Can you work these out from the model? Positions are in its coordinate system, mm. A direction names the side the tool comes from. Give positions to 0.01 mm unless a question says otherwise; leave off trailing zeros. Write each loop counter-clockwise with the first axis right and the second up, starting at its lowest first coordinate (ties: lowest second). Pieces come first, ordered by that corner, then holes.
1. On a 3-axis mill with a long thin cutter (end or side, diameter ignored), from which of +Z, -Z, +X, -X, +Y, -Y can I reach the whole of each face in a straight line? I mean faces 4 (the flat face through (0, 0, 62.5)), 5 (the flat face through (22.424, 11.39, -7.5)), 6 (the flat face through (9, 9, 12.5)). Say none if no direction works.
2. Suppose I cut it at C-C (z = 4). Please give me the cut outline in (x, y), and give its area (3 significant figures).
3. If I drill on probe 1 along Y at (x, z) = (-3, -4); probe 2 along Y at (x, z) = (-17, -4.5); probe 3 along Z at (x, y) = (2, 18), over which ranges is the centre line in solid material (lowest first)?
4. Suppose I cut it at A-A (x = 0). Please give me the cut outline in (y, z).
5. I'm going to push flat-ended pins straight in: pin 1 (1.5 mm diameter, centred on y = -22.5, z = -1.5, fed in from -X); pin 2 (1 mm diameter, centred on x = -24, y = 2.5, fed in from +Z); pin 3 (3 mm diameter, centred on y = -1, z = 3.5, fed in from -X); pin 4 (12 mm diameter, centred on y = -11, z = 38, fed in from -X). Where does each tip first touch, or does it pass through?
6. Suppose I cut it at D-D (z = 18). Please give me the cut outline in (x, y).
7. Thinking about a two-plate mould opening in Y: for faces 1 (the flat face through (0, 0, -12.5)), 2 (the cylindrical face through (11.923, 3.755, 34.685)), 3 (the cylindrical face through (-4.336, -19.524, 7.57)), which applies, pulls with the +Y half, pulls with the -Y half, needs draft (parallel to the pull), parting line crosses it, or undercut?
```python
from build123d import *

# Parameters (mm, degrees)
F0_R     = 30.360351
F0_R_2   = 20
F1_DEPTH = 7.5
F2_R     = 5
F3_R     = 5
F4_R     = 5
F5_DEPTH = 12.5
F6_R     = 12.5
F7_DEPTH = 50
F8_R     = 5


with BuildPart() as f1:
    # F0 (on Top) → F1 (new body, symmetric)
    with BuildSketch(Plane.XY):
        Circle(F0_R)
        Circle(F0_R_2, mode=Mode.SUBTRACT)
    extrude(amount=F1_DEPTH, both=True)

    # F2
    f2_edges = [f1.edges().sort_by_distance(p)[0] for p in [
        (-30.360351, 0, -7.5),
        (-20, 0, -7.5),
    ]]
    fillet(f2_edges, radius=F2_R)

    # F3
    f3_edges = [f1.edges().sort_by_distance(p)[0] for p in [
        (-20, 0, 7.5),
    ]]
    fillet(f3_edges, radius=F3_R)

    # F4
    f4_edges = [f1.edges().sort_by_distance(p)[0] for p in [
        (-30.360351, 0, 7.5),
    ]]
    fillet(f4_edges, radius=F4_R)

    # F0 (on Top) → F5 (join, symmetric)
    with BuildSketch(Plane.XY):
        Circle(F0_R_2)
    extrude(amount=F5_DEPTH, both=True)

    # F6 (on face) → F7 (join)
    with BuildSketch(Plane.XY.offset(12.5)):
        Circle(F6_R)
    extrude(amount=F7_DEPTH)

    # F8
    f8_edges = [f1.edges().sort_by_distance(p)[0] for p in [
        (-12.5, 0, 62.5),
    ]]
    fillet(f8_edges, radius=F8_R)


solid = f1.part
```
Checks:
1. face 4: +Z, +X, -X, +Y, -Y
1. face 5: -Z
1. face 6: +Z
2. outline: circle Ø60.26 at (0, 0); circle Ø40 at (0, 0); hole circle Ø40.46 at (0, 0)
2. area: 2,820 mm2
3. probe 1: y = -29.98 to -20.01, -19.77 to 19.77, 20.01 to 29.98
3. probe 2: y = -24.65 to -11.31, -10.54 to 10.54, 11.31 to 24.65
3. probe 3: z = -12.5 to 12.5
4. outline: (-30.36, -2.5) arc R5 ccw to (-25.36, -7.5) - (-25, -7.5) arc R5 ccw to (-20, -2.5) - (-20, -12.5) - (20, -12.5) - (20, -2.5) arc R5 ccw to (25, -7.5) - (25.36, -7.5) arc R5 ccw to (30.36, -2.5) - (30.36, 2.5) arc R5 ccw to (25.36, 7.5) - (25, 7.5) arc R5 ccw to (20, 2.5) - (20, 12.5) - (12.5, 12.5) - (12.5, 57.5) arc R5 ccw to (7.5, 62.5) - (-7.5, 62.5) arc R5 ccw to (-12.5, 57.5) - (-12.5, 12.5) - (-20, 12.5) - (-20, 2.5) arc R5 ccw to (-25, 7.5) - (-25.36, 7.5) arc R5 ccw to (-30.36, 2.5) - close
5. pin 1: stops at x = -21.18
5. pin 2: stops at z = 7.49
5. pin 3: stops at x = -30.36
5. pin 4: stops at x = -11.46
6. outline: circle Ø25 at (0, 0)
7. face 1: needs draft
7. face 2: parting line crosses it
7. face 3: undercut
